Autodesk Inventor part; units mm, degrees
ref_plane "YZ Plane" through (0, 0, 0) normal (1, 0, 0) x (0, 1, 0)
ref_plane "XZ Plane" through (0, 0, 0) normal (0, 1, 0) x (-1, 0, 0)
ref_plane "XY Plane" through (0, 0, 0) normal (0, 0, 1) x (1, 0, 0)
sketch "Sketch1" plane through (0, 0, 0) normal (0, 0, 1) x (1, 0, 0)
  circle A0 centre (0, 0) radius 23.8125
  circle A1 centre (0, 0) radius 36.5125
  line L0 (36.5125, -165.1) -> (-14.2875, -165.1) construction
  line L1 (36.5125, 0) -> (36.5125, -165.1)
  line L2 (-36.1762, -4.9442) -> (-14.2875, -165.1) construction
  line L3 (36.5125, -44.45) -> (-14.2875, -44.45) construction
  line L4 (-14.2875, -44.45) -> (-14.2875, -431.8) construction
  line L5 (-14.2875, -431.8) -> (36.5125, -431.8) construction
  line L6 (36.5125, -431.8) -> (36.5125, -44.45) construction
  line L7 (8.7327, -97.2312) -> (-152.2848, -442.5345) construction
  line L8 (-152.2848, -442.5345) -> (-175.3051, -431.8) construction
  line L9 (-175.3051, -431.8) -> (-14.2875, -86.4967) construction
  line L10 (-14.2875, -86.4967) -> (8.7327, -97.2312) construction
  line L11 (36.5125, -431.8) -> (11.1125, -431.8) construction
  line L12 (11.1125, -431.8) -> (11.1125, -501.65) construction
  line L13 (11.1125, -501.65) -> (36.5125, -501.65) construction
  line L14 (36.5125, -501.65) -> (36.5125, -431.8) construction
  line L15 (-150.8125, -431.8) -> (-150.8125, -501.65) construction
  line L16 (-2.7774, -91.864) -> (-19.4192, -127.5524) construction
  line L17 (-36.3765, 3.1489) -> (-36.3765, -165.1) construction
  line L18 (-50.9408, -165.1) -> (36.5125, -165.1)
  line L19 (-50.9408, -165.1) -> (-36.3765, 3.1489)
  line L20 (-50.9408, -165.1) -> (-14.2875, -86.4967)
  line L21 (-14.2875, -44.45) -> (-14.2875, -86.4967)
  line L22 (-14.2875, -44.45) -> (-30.4024, -20.2202)
  point P0 (23.8125, -431.8)
  point P1 (-8.1446, -103.3741)
  point P2 (23.8125, -57.15)
  point P3 (11.1125, -57.15)
  point P4 (-1.5875, -57.15)
  point P5 (11.1125, -44.45)
  point P6 (-13.5119, -114.8842)
  point P7 (-18.8791, -126.3943)
  point P8 (-24.2464, -137.9044)
  point P9 (-29.6137, -149.4145)
  dimension "d0" = 47.625
  dimension "d1" = 12.7
  dimension "d2" = 50.8
  dimension "d3" = 165.1
  dimension "d4" = 50.8
  dimension "d5" = 387.35
  dimension "d6" = 25.4
  dimension "d7" = 25
  dimension "d8" = 381
  dimension "d10" = 25.4
  dimension "d11" = 69.85
  dimension "d13" = 431.8
  dimension "d15" = 187.325
  dimension "d17" = 12.7
  dimension "d18" = 12.7
  dimension "d19" = 12.7
  dimension "d20" = 12.7
  dimension "d23" = 12.7
extrude "Extrusion1" add sketch "Sketch1" against normal blind 6.35 contours A1 | L1 L18 L20 L21 L22 A1
hole "Hole1" at (23.8125, -57.15, 0) at (11.1125, -57.15, 0) at (-1.5875, -57.15, 0) at (-18.8791, -126.3943, 0) at (-24.2464, -137.9044, 0) at (-29.6137, -149.4145, 0) direction (0, 0, -1) diameter 6.604 end through all
sketch "Sketch2" plane through (0, 0, -6.35) normal (0, 0, -1) x (-1, 0, 0)
  circle A0 centre (0, 0) radius 23.8125
  circle A1 centre (0, 0) radius 17.4625
  dimension "d37" = 6.35
extrude "Extrusion2" add sketch "Sketch2" against normal blind 3.175
sketch "Sketch3" plane through (0, 0, 0) normal (0, 0, 1) x (1, 0, 0)
  circle A0 centre (-24.2464, -137.9044) radius 3.302 construction
  circle A1 centre (-1.5875, -57.15) radius 3.302 construction
  circle A2 centre (23.8125, -57.15) radius 3.302 construction
  circle A3 centre (11.1125, -57.15) radius 3.302 construction
  circle A4 centre (-18.8791, -126.3943) radius 3.302 construction
  circle A5 centre (-29.6137, -149.4145) radius 3.302 construction
  circle A6 centre (0, 0) radius 23.8125 construction
  line L0 (36.5125, 0) -> (36.5125, -165.1) construction
  line L1 (36.5125, -165.1) -> (-50.9408, -165.1) construction
  circle A7 centre (-24.2464, -137.9044) radius 3.302 construction
  circle A8 centre (-1.5875, -57.15) radius 3.302 construction
  circle A9 centre (23.8125, -57.15) radius 3.302 construction
  circle A10 centre (11.1125, -57.15) radius 3.302 construction
  circle A11 centre (-18.8791, -126.3943) radius 3.302 construction
  circle A12 centre (-29.6137, -149.4145) radius 3.302 construction
  circle A13 centre (0, 0) radius 23.8125 construction
  line L2 (36.5125, 0) -> (36.5125, -165.1) construction
  line L3 (36.5125, -165.1) -> (-50.9408, -165.1) construction
  line L4 (-175.3051, -431.8) -> (-14.2875, -86.4967) construction
  line L5 (8.7327, -97.2312) -> (-152.2848, -442.5345) construction
  line L6 (-14.2875, -44.45) -> (-14.2875, -431.8) construction
  line L7 (-14.2875, -86.4967) -> (-14.2875, -44.45)
  line L8 (-14.2875, -44.45) -> (-30.4024, -20.2202)
  arc A14 (36.5125, 0) -> (-30.4024, -20.2202) centre (0, 0) ccw
  line L9 (-50.9408, -165.1) -> (-14.2875, -86.4967)
  line L10 (-14.2875, -86.4967) -> (-14.2875, -44.45)
  line L11 (-14.2875, -44.45) -> (-30.4024, -20.2202)
  arc A15 (36.5125, 0) -> (-30.4024, -20.2202) centre (0, 0) ccw
  line L12 (-50.9408, -165.1) -> (-14.2875, -86.4967)
fillet "Fillet1" radius 3.175 4 edges at (-14.2875, -44.45, -3.175) (-14.2875, -86.4967, -3.175) (-50.9408, -165.1, -3.175) (36.5125, -165.1, -3.175)
properties part number "CL7-007" material "Aluminum 6061"
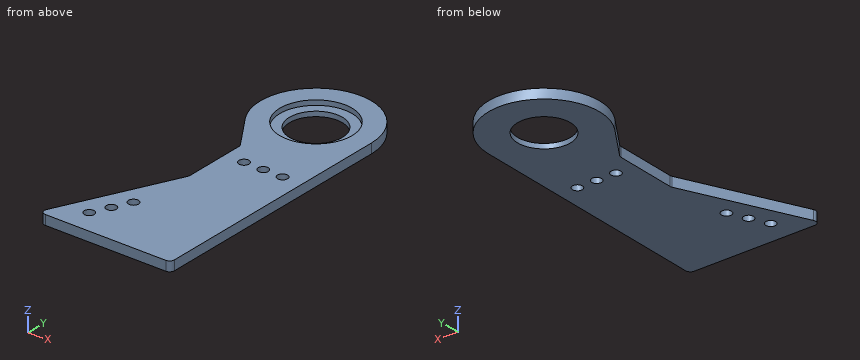
The model under review builds one solid part; all positions refer to its coordinate system, in mm. Give positions to 0.01 mm unless a question says otherwise; leave off trailing zeros. Loops run counter-clockwise (first coordinate to the right, second up) from the corner with the lowest first, then second, coordinate; pieces in that order, holes last. Notation, with made-up numbers: (77, -34.75) -> (91, -34.75) arc R31 cw to (91, 3.25) -> close; hole circle Ø5 at (-33, -36.75). An arc over 180 degrees is marked (long way). Put each result on its own line as item: value. Start each with the question number.
1. We need section A-A on y = -57.15. State the section outline as (x, z) points, then the cut area to 3 significant figures.
2. Clearance check with flat-ended pins moving along their axes: P1, Ø5.5, axis at x = -1.59, y = -57.15, coming from the +Z side; P2, Ø2, axis at y = -6.5, z = -3.5, coming from the -X side; P3, Ø2, axis at x = 5, z = -4.5, coming from the +Y side; P4, Ø5, axis at x = -7.5, y = -18, coming from the +Z side (3 decimals). State where each tip first meets the part, or that it passes through.
3. We need section B-B on x = -7.5. State the section outline as (y, z) points (3 decimals).
4. We need section C-C on z = -1.75. State how many separate pieces and enclosed holes the cut face has, then the cut area to 3 significant figures.
5. We need section D-D on y = -149. State the section outline as (x, z) points, then the cut area to 3 significant figures.
6. Wall thickness on probe 1 along X at (y, z) = (-57.15, -4.5); probe 2 along Y at (x, z) = (-29, -0.5); probe 3 along Y at (x, z) = (-27, -2): over which ranges is each line inside the solid? List them lowest first.
Determined:
1. outline: (-14.29, -6.35) -> (-4.89, -6.35) -> (-4.89, 0) -> (-14.29, 0) -> close; (1.71, -6.35) -> (7.81, -6.35) -> (7.81, 0) -> (1.71, 0) -> close; (14.41, -6.35) -> (20.51, -6.35) -> (20.51, 0) -> (14.41, 0) -> close; (27.11, -6.35) -> (36.51, -6.35) -> (36.51, 0) -> (27.11, 0) -> close
1. area: 197 mm^2
2. P1: through
2. P2: x = -36.1
2. P3: y = 36.29
2. P4: z = -3.175
3. outline: (-165.1, -6.35) -> (-15.77, -6.35) -> (-15.77, -3.175) -> (-22.601, -3.175) -> (-22.601, 0) -> (-165.1, 0) -> close; (15.77, -6.35) -> (35.734, -6.35) -> (35.734, 0) -> (22.601, 0) -> (22.601, -3.175) -> (15.77, -3.175) -> close
4. separate pieces: 1
4. enclosed holes: 7
4. area: 10,500 mm^2
5. outline: (-43.43, -6.35) -> (-32.89, -6.35) -> (-32.89, 0) -> (-43.43, 0) -> close; (-26.34, -6.35) -> (36.51, -6.35) -> (36.51, 0) -> (-26.34, 0) -> close
5. area: 466 mm^2
6. probe 1: -14.29 to -4.89, 1.71 to 7.81, 14.41 to 20.51, 27.11 to 36.51
6. probe 2: -165.1 to -152.66, -146.17 to -118.05, -22.33 to 22.18
6. probe 3: -165.1 to -151.43, -147.4 to -139.73, -136.08 to -113.76, -25.34 to 24.58
